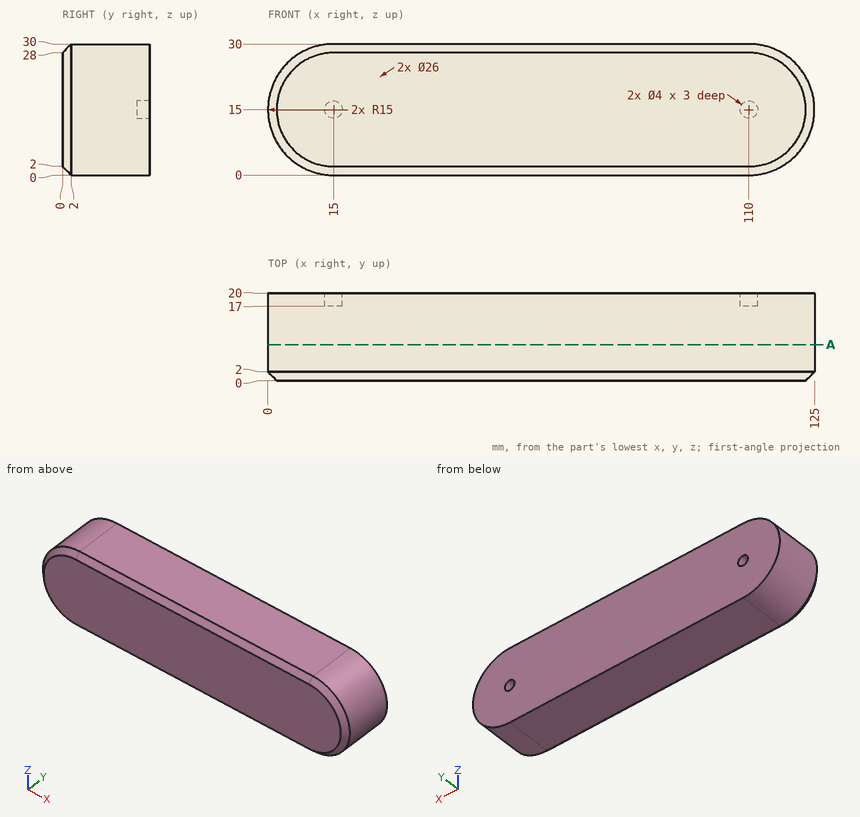
Print and shaded views of the part. All mm, measured from the part's lowest x, y and z. Give positions to 0.01 mm unless a question says otherwise; leave off trailing zeros. Loops run counter-clockwise (first coordinate to the right, second up) from the corner with the lowest first, then second, coordinate; pieces in that order, holes last. Notation, with made-up numbers: (-37, 19.5) - (21, 19.5) arc R16 ccw to (21, 38.5) - close; hole circle Ø10 at (53, 51). An arc over 180 degrees is marked (long way). Use a Markdown table: item, result.
(1) Wall check: line 1 along X through (y, z) = (18.85, 15); line 2 along Z through (x, y) = (110, 19.3); line 3 along X through (y, z) = (18, 17.5). Give the ranges that are in metal, low to high.
Taken from the geometry:
| item | result |
|---|---|
| line 1 | 0 to 13, 17 to 108, 112 to 125 |
| line 2 | 0 to 13, 17 to 30 |
| line 3 | 0.21 to 124.79 |
(2) Drop flat-ended pins along their axis: pin 1 Ø4.5 at (x, z) = (110, 15) entering from +Y; pin 2 Ø4 at (y, z) = (12.5, 7.5) entering from +X; pin 3 Ø3 at (x, z) = (15, 15) entering from +Y; pin 4 Ø4 at (y, z) = (6, 20.5) entering from +X. Give the stop position or say it passes through.
Taken from the geometry:
| item | result |
|---|---|
| pin 1 | y = 20 |
| pin 2 | x = 123.96 |
| pin 3 | y = 17 |
| pin 4 | x = 124.59 |
(3) Band-saw the part on A-A (y = 8.25). Give the cut face in (x, z), and give its area (3 significant figures).
Taken from the geometry:
| item | result |
|---|---|
| outline | (15, 0) - (110, 0) arc R15 ccw to (110, 30) - (15, 30) arc R15 ccw to start |
| area | 3,560 mm2 |
